Can you work these out from the drawing? Everything is in mm from the part's minimum corner. A direction names the side the tool comes from. Round coordinates to 2 decimals unless told otherwise and drop trailing zeros. Write each loop counter-clockwise with the first axis right and the second up, starting at its lowest first coordinate (ties: lowest second). Pieces come first, ordered by that corner, then holes. Notation, with made-up numbers: (-6, 15) -> (18, 15) arc R23 cw to (18, 33) -> close; hole circle Ø7 at (80, -14.75). An arc over 180 degrees is marked (long way). Put each result on its own line as item: value. Start each with the question number.
1. Suppose I cut it at A-A (y = 54). Please give me the cut outline in (x, z).
2. Suppose I cut it at B-B (z = 51.5). Please give me the cut outline in (x, y), then the cut area to 3 significant figures.
3. For pin 1 (10 mm diameter, centred on y = 9.5, z = 42.5, fed in from -X); pin 2 (2 mm diameter, centred on x = 33, z = 47.5, fed in from +Y); pin 3 (1.5 mm diameter, centred on x = 47, y = 14.5, fed in from -Z); pin 4 (2 mm diameter, centred on x = 28, y = 17, fed in from -Z), each with a flat end and sliding along its axis, tell me the tip position at first contact or that it passes through.
4. Suppose I cut it at D-D (y = 40). Please give me the cut outline in (x, z).
5. I need wall thicknesses on probe 1 along Z at (x, y) = (36, 9); probe 2 along X at (y, z) = (29.5, 54); probe 3 along X at (y, z) = (21, 36.5). Which ranges of each line are inside material? Lowest first, please. Write a range as from..to.
6. Suppose I cut it at C-C (x = 25). Please give me the cut outline in (y, z).
7. We'd pull the mould along Z, two halves only. Please class the marked faces 3, 4, 5 and 6: +Z half, -Z half, draft (parallel to the pull), parting line (faces both ways), or undercut.
8. Which directions (+Z, -Z, +X, -X, +Y, -Y) give clear straight access to the entire face, cutting with the end or side of a thin tool? Please do the marked faces 1 and 2.
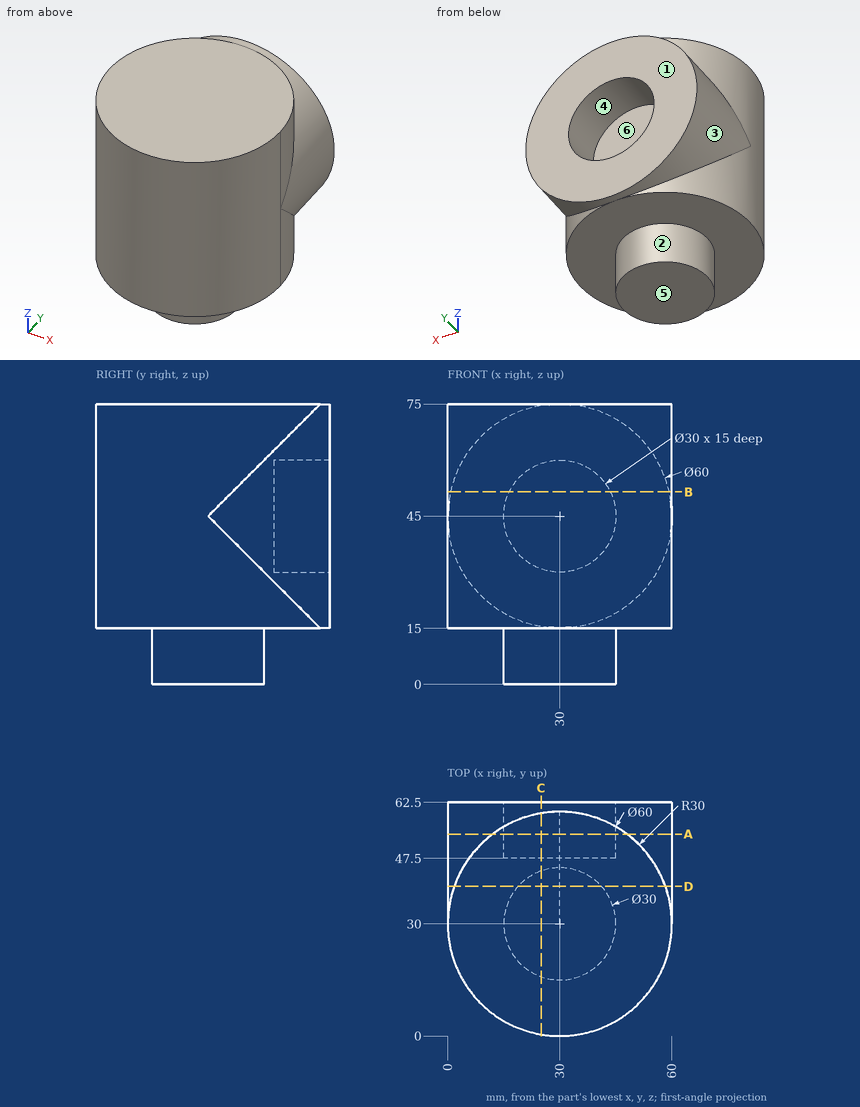
Verdict:
1. outline: (12, 15) -> (48, 15) -> (48, 21) arc R30 ccw to (48, 69) -> (48, 75) -> (12, 75) -> (12, 69) arc R30 ccw to (12, 21) -> close; hole circle Ø30 at (30, 45)
2. outline: (0.71, 36.5) arc R30 ccw (long way) to (59.29, 36.5) -> (59.29, 62.5) -> (43.52, 62.5) -> (43.52, 47.5) -> (16.48, 47.5) -> (16.48, 62.5) -> (0.71, 62.5) -> close
2. area: 2,920 mm^2
3. pin 1: stops at x = 4.31
3. pin 2: stops at y = 47.5
3. pin 3: stops at z = 15
3. pin 4: stops at z = 0
4. outline: (1.72, 15) -> (18.82, 15) -> (18.82, 0) -> (41.18, 0) -> (41.18, 15) -> (58.28, 15) -> (58.28, 35) arc R30 ccw to (58.28, 55) -> (58.28, 75) -> (1.72, 75) -> (1.72, 55) arc R30 ccw to (1.72, 35) -> close
5. probe 1: z = 15..75
5. probe 2: x = 0..60
5. probe 3: x = 1.38..58.62
6. outline: (0.42, 15) -> (15.86, 15) -> (15.86, 0) -> (44.14, 0) -> (44.14, 15) -> (59.58, 15) -> (59.58, 15.42) -> (62.5, 15.42) -> (62.5, 30.86) -> (47.5, 30.86) -> (47.5, 59.14) -> (62.5, 59.14) -> (62.5, 74.58) -> (59.58, 74.58) -> (59.58, 75) -> (0.42, 75) -> close
7. face 3: parting line
7. face 4: undercut
7. face 5: -Z half
7. face 6: undercut
8. face 1: +Z, -Z, +X, -X, +Y
8. face 2: -Z
